The listing builds one solid part. Answer for the finished solid, in the listing's coordinates (mm). Face numbers are marked on the shaded views. Coordinates: 2 decimals unless noted, no trailing zeros. Write each loop counter-clockwise with the first axis right and the second up, starting at its lowest first coordinate (ties: lowest second). Pieces come first, ordered by that corner, then holes. Notation, with made-up numbers: M 87.25,83 L 129.25,83 A15 cw 129.25,96 Z; hole C -27.75,15 d8. An arc over 180 degrees is marked long. Put each result on its own line as item: value. Start each with the question number.
```python
from build123d import *

# Parameters (mm, degrees)
BOX002_W      = 20
BOX002_H      = 30
BOX002_DEPTH  = 2
FILLET003_R   = 3
BOX001_W      = 40
BOX001_H      = 30
BOX001_DEPTH  = 2
FILLET002_R   = 3
BOX_W         = 100
BOX_H         = 50
BOX_DEPTH     = 2
FILLET_R      = 2
FILLET001_R   = 3
BOX003_W      = 30
BOX003_H      = 2
BOX003_DEPTH  = 20
FILLET004_R   = 3
ARRAY_Y_COUNT = 2
ARRAY_Y_PITCH = 48


with BuildPart() as fillet003:
    # Box002 → Box002 (new body)
    with BuildSketch(Plane.XY):
        with Locations((10, 15)):
            Rectangle(BOX002_W, BOX002_H)
    extrude(amount=BOX002_DEPTH)

    # Fillet003
    fillet003_edges = [fillet003.edges().sort_by_distance(p)[0] for p in [
        (0, 0, 1),
        (0, 30, 1),
        (20, 0, 1),
        (20, 30, 1),
    ]]
    fillet(fillet003_edges, radius=FILLET003_R)


with BuildPart() as fillet003_1:
    # Fillet003 placement: moved
    add(fillet003.part.moved(Location((70, 10, 0))))


with BuildPart() as fillet002:
    # Box001 → Box001 (new body)
    with BuildSketch(Plane(origin=(10, 10, 0), x_dir=(1, 0, 0), z_dir=(0, 0, 1))):
        with Locations((20, 15)):
            Rectangle(BOX001_W, BOX001_H)
    extrude(amount=BOX001_DEPTH)

    # Fillet002
    fillet002_edges = [fillet002.edges().sort_by_distance(p)[0] for p in [
        (10, 10, 1),
        (10, 40, 1),
        (50, 10, 1),
        (50, 40, 1),
    ]]
    fillet(fillet002_edges, radius=FILLET002_R)


with BuildPart() as cut001:
    # Box → Box (new body)
    with BuildSketch(Plane.XY):
        with Locations((50, 25)):
            Rectangle(BOX_W, BOX_H)
    extrude(amount=BOX_DEPTH)

    # Fillet
    fillet_edges = [cut001.edges().sort_by_distance(p)[0] for p in [
        (0, 0, 1),
        (0, 50, 1),
        (100, 0, 1),
    ]]
    fillet(fillet_edges, radius=FILLET_R)

    # Fillet001
    fillet001_edges = [cut001.edges().sort_by_distance(p)[0] for p in [
        (100, 50, 1),
    ]]
    fillet(fillet001_edges, radius=FILLET001_R)

    # Cut: cut Fillet002
    add(fillet002.part, mode=Mode.SUBTRACT)

    # Cut001: cut Fillet003
    add(fillet003_1.part, mode=Mode.SUBTRACT)


with BuildPart() as fusion:
    # Box003 → Box003 (new body)
    with BuildSketch(Plane.XY):
        with Locations((15, 1)):
            Rectangle(BOX003_W, BOX003_H)
    extrude(amount=BOX003_DEPTH)

    # Fillet004
    fillet004_edges = [fusion.edges().sort_by_distance(p)[0] for p in [
        (0, 1, 20),
        (30, 1, 20),
    ]]
    fillet(fillet004_edges, radius=FILLET004_R)

    # Array Y: Fusion ×2


with BuildPart() as fusion_1:
    add(fusion.part)
    with Locations(*[(0, i * ARRAY_Y_PITCH, 0) for i in range(1, ARRAY_Y_COUNT)]):
        add(fusion.part)

    # Fusion: union Cut001
    add(cut001.part)


solid = fusion_1.part
```
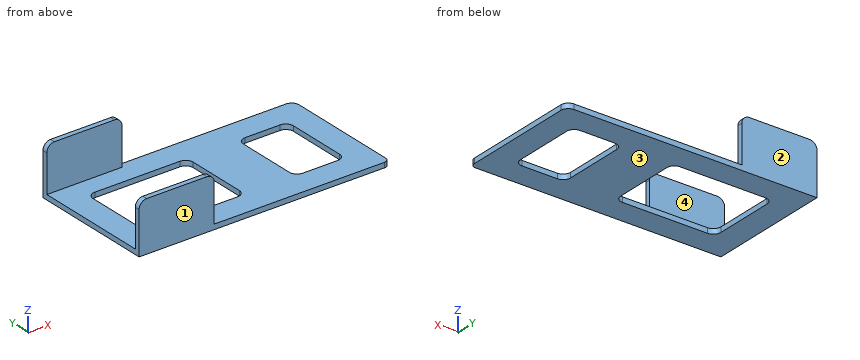
1) A cutting plane is placed at D-D on x = 8. Write down the section's boundary in (y, z), then the cut area to 3 significant figures.
2) A cutting plane is placed at B-B on z = 7.25. Write down the section's boundary in (x, y).
3) Given pin 1 Ø25 at (x, y) = (31, 29.5) entering from +Z; pin 2 Ø1 at (y, z) = (49.5, 9.5) entering from +X, each flat-ended and moving along its own axis, determine where each tip first touches the part or whether it passes through.
4) Straight lines are drawn through the part: probe 1 along Y at (x, z) = (25, 9.5); probe 2 along Z at (x, y) = (33, 9.5). For each, find the intervals that lie inside material, in ascending order.
5) Determine the mould class of the marked faces 1, 2, 3 and 4 for opening direction Y: +Y half, -Y half, draft (parallel to the pull), parting line (faces both ways), or undercut.
6) A cutting plane is placed at C-C on x = 84. Write down the section's boundary in (y, z).
7) A cutting plane is placed at A-A on y = 33.5. Write down the section's boundary in (x, z), then the cut area to 3 significant figures.
Answers follow:
1. outline: M 0,0 L 50,0 L 50,20 L 48,20 L 48,2 L 2,2 L 2,20 L 0,20 Z
1. area: 172 mm²
2. outline: M 0,0 L 30,0 L 30,2 L 0,2 Z; M 0,48 L 30,48 L 30,50 L 0,50 Z
3. pin 1: stops at z = 2
3. pin 2: stops at x = 30
4. probe 1: y = 0 to 2, 48 to 50
4. probe 2: z = 0 to 2
5. face 1: -Y half
5. face 2: +Y half
5. face 3: draft
5. face 4: undercut
6. outline: M 0,0 L 10,0 L 10,2 L 0,2 Z; M 40,0 L 50,0 L 50,2 L 40,2 Z
7. outline: M 0,0 L 10,0 L 10,2 L 0,2 Z; M 50,0 L 70,0 L 70,2 L 50,2 Z; M 90,0 L 100,0 L 100,2 L 90,2 Z
7. area: 80.0 mm²
